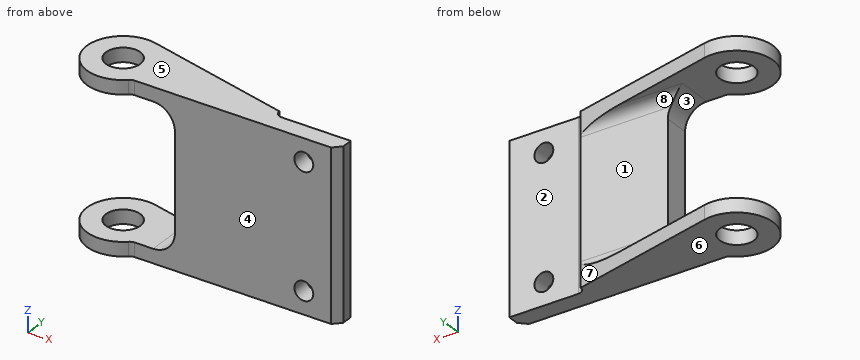
Autodesk Inventor part; units mm, degrees
ref_plane "YZ Plane" through (0, 0, 0) normal (1, 0, 0) x (0, 1, 0)
ref_plane "XZ Plane" through (0, 0, 0) normal (0, 1, 0) x (-1, 0, 0)
ref_plane "XY Plane" through (0, 0, 0) normal (0, 0, 1) x (1, 0, 0)
sketch "Sketch1" plane through (0, 0, 0) normal (0, 0, 1) x (1, 0, 0)
  arc A0 (2.3256, 9.7258) -> (7.1414, -7) centre (0, 0) ccw
  line L0 (7.1414, -7) -> (64, -7)
  line L1 (64, -7) -> (64, -2)
  line L2 (64, -2) -> (45, -2)
  arc A1 (43, 0) -> (45, -2) centre (45, 0) ccw
  line L3 (43, 0) -> (2.3256, 9.7258)
  dimension "d0" = 20
  dimension "d1" = 21
  dimension "d2" = 64
  dimension "d3" = 5
  dimension "d4" = 2
  dimension "d5" = 7
extrude "Extrusion1" add sketch "Sketch1" along normal mid plane 46.5
sketch "Sketch2" plane through (0, 0, 23.25) normal (0, 0, 1) x (1, 0, 0)
  arc A0 (2.3256, 9.7258) -> (7.1414, -7) centre (0, 0) ccw
hole "Hole1" at (0, 0, 23.25) direction (0, 0, -1) diameter 9.5 depth 46.5
sketch "Sketch4" plane through (64, -7, 23.25) normal (1, 0, 0) x (0, 0, -1)
  line L0 (46.5, 17) -> (0, 17)
  line L1 (46.5, 7) -> (0, 7)
  line L2 (3.85, 17) -> (42.65, 17)
  line L3 (42.65, 17) -> (42.65, 10)
  line L4 (39.65, 7) -> (6.85, 7)
  line L5 (3.85, 10) -> (3.85, 17)
  arc A0 (3.85, 10) -> (6.85, 7) centre (6.85, 10) ccw
  arc A1 (39.65, 7) -> (42.65, 10) centre (39.65, 10) ccw
  point P0 (23.25, 7)
  point P1 (23.25, 7)
  dimension "d20" = 38.8
  dimension "d21" = 3
extrude "Extrusion3" cut sketch "Sketch4" against normal up to next
sketch "Sketch6" plane through (0, 0, 0) normal (0, 1, 0) x (-1, 0, 0)
  line L0 (10, 16.4) -> (10, -16.4)
  line L1 (-2.3256, -19.4) -> (-30.4537, -19.4)
  line L2 (-30.4537, 19.4) -> (-2.3256, 19.4)
  line L3 (10, -19.4) -> (-13, -19.4)
  line L4 (-19, -13.4) -> (-19, 13.4)
  line L5 (-13, 19.4) -> (10, 19.4)
  line L6 (10, 19.4) -> (10, -19.4)
  arc A0 (-19, -13.4) -> (-13, -19.4) centre (-13, -13.4) ccw
  arc A1 (-13, 19.4) -> (-19, 13.4) centre (-13, 13.4) ccw
  point P0 (0, 0)
  point P1 (-19, -19.4)
  point P2 (10, 0)
  point P3 (-13, -19.4)
  point P4 (-2.3256, 19.4)
  point P5 (-13, 19.4)
  dimension "d24" = 38.8
  dimension "d26" = 6
  dimension "d29" = 19
extrude "Extrusion4" cut sketch "Sketch6" along normal through all both and the other way through all
sketch "Sketch7" plane through (45, -2, 23.25) normal (0, 1, 0) x (1, 0, 0)
  line L0 (19, 46.5) -> (19, 0)
  line L1 (9.5, 40.25) -> (9.5, 6.25) construction
  line L2 (19, 46.5) -> (19, 0) construction
  point P0 (-45, 23.25)
  point P1 (9.5, 23.25)
  dimension "d31" = 34
  dimension "d33" = 9.5
hole "Hole2" at (54.5, -2, 17) at (54.5, -2, -17) direction (0, -1, 0) diameter 5.2 end through all
chamfer "Chamfer1" distance 2 angle 45 1 edges at (64, -7, 0)
fillet "Fillet1" radius 2 2 edges at (7.1414, -7, 21.325) (7.1414, -7, -21.325)
properties material "Stainless Steel"
Can you work these out from the model? Positions are in its coordinate system, mm. Face numbers are marked on the shaded views. A direction names the side the tool comes from. Give positions to 0.01 mm unless a question says otherwise; leave off trailing zeros. Loops run counter-clockwise (first coordinate to the right, second up) from the corner with the lowest first, then second, coordinate; pieces in that order, holes last. Notation, with made-up numbers: M 58,-39.75 L 80,-39.75 A25 ccw 80,-20.75 Z; hole C 56.25,-0.5 d1. An arc over 180 degrees is marked long. Use CSV: the item, a comma, the result in double quotes. Start each with the question number.
1. Imagine slicing it at A-A, the plane x = 54.5. Write out the boundary of the cut face in (y, z).
2. Imagine slicing it at B-B, the plane y = -3.75. Write out the boundary of the cut face in (x, z).
3. If we mould it in two halves opening along Z, with no side actions, what happens to the marked faces 6, 7 and 8? For each: released by +Z, released by -Z, zero draft, split by the parting line, or undercut.
4. Imagine slicing it at D-D, the plane y = 6. Write out the boundary of the cut face in (x, z), plus the area to 3 significant figures.
5. If I drill on L1, parallel to Z at x = 7.5, y = 7.25; L2, parallel to Z at x = 54.5, y = -5.6; L3, parallel to Y at x = 0, z = 22.4, over which ranges is the centre line in solid material (lowest first)?
6. Imagine slicing it at C-C, the plane x = 0. Write out the boundary of the cut face in (y, z).
7. On a 3-axis mill with a long thin cutter (end or side, diameter ignored), from which of +Z, -Z, +X, -X, +Y, -Y can I reach the whole of each face in a straight line? I mean the marked faces 1, 2, 3, 4 and 5. Say none if no direction works.
8. For P1, Ø20, axis at x = 30, z = 7, coming from the +Y side; P2, Ø2, axis at y = -1, z = 16.5, coming from the -X side; P3, Ø9.5, axis at x = 50, z = -11.5, coming from the +Y side, each with a flat end and sliding along its axis, tell me the tip position at first contact or that it passes through.
Response values:
1,outline,"M -7,-23.25 L -2,-23.25 L -2,-19.6 L -7,-19.6 Z; M -7,-14.4 L -2,-14.4 L -2,14.4 L -7,14.4 Z; M -7,19.6 L -2,19.6 L -2,23.25 L -7,23.25 Z"
2,outline,"M -9.27,-23.25 L -2.92,-23.25 L -2.92,-19.4 L -9.27,-19.4 Z; M -9.27,19.4 L -2.92,19.4 L -2.92,23.25 L -9.27,23.25 Z; M 2.92,-23.25 L 64,-23.25 L 64,23.25 L 2.92,23.25 L 2.92,19.4 L 13,19.4 A6 cw 19,13.4 L 19,-13.4 A6 cw 13,-19.4 L 2.92,-19.4 Z; hole C 54.5,-17 d5.2; hole C 54.5,17 d5.2"
3,face 6,"released by -Z"
3,face 7,"zero draft"
3,face 8,"undercut"
4,outline,"M -8,-23.25 L 17.91,-23.25 L 17.91,-19.4 L -8,-19.4 Z; M -8,19.4 L 17.91,19.4 L 17.91,23.25 L -8,23.25 Z"
4,area,"199 mm^2"
5,L1,"-23.25 to -19.4, 19.4 to 23.25"
5,L2,"-23.25 to -19.6, -14.4 to 14.4, 19.6 to 23.25"
5,L3,"-10 to -4.75, 4.75 to 10"
6,outline,"M -10,-23.25 L -4.75,-23.25 L -4.75,-19.4 L -10,-19.4 Z; M -10,19.4 L -4.75,19.4 L -4.75,23.25 L -10,23.25 Z; M 4.75,-23.25 L 10,-23.25 L 10,-19.4 L 4.75,-19.4 Z; M 4.75,19.4 L 10,19.4 L 10,23.25 L 4.75,23.25 Z"
7,face 1,"+X, -X, +Y"
7,face 2,"+Z, -Z, +X, +Y"
7,face 3,"-X, +Y, -Y"
7,face 4,"+Z, -Z, +X, -Y"
7,face 5,"+Z, +X, -X, +Y, -Y"
8,P1,"y = 0.06"
8,P2,"x = 17.38"
8,P3,"y = -2"
